Build history of the part. All positions in model axes, mm. A direction names the side the tool comes from. Coordinates: 2 decimals unless noted, no trailing zeros.
(1) Flat gauge pins, fed straight in: P1, Ø6, axis at x = 438, y = 715.5, coming from the -Z side; P2, Ø6.5, axis at x = 301, y = 824.5, coming from the +Z side. Where does each tip first touch, or does it go through?
(2) Wall check: L1, parallel to X at y = 823.5, z = 10. Give the ranges that are in metal, low to high.
(3) Tool access for faces 1 (the face through (296, 685.625, 6)), 2 (the face through (300, 809, 7.7)): list every direction of +Z, -Z, +X, -X, +Y, -Y with a clear straight run to the whole face (end or side of a thin tool).
from build123d import *

# Parameters (mm, degrees)
SKETCH002_W     = 600
SKETCH002_H     = 250
PAD002_DEPTH    = 12.7
SKETCH008_W     = 13
SKETCH008_H     = 264.944031
POCKET002_DEPTH = 5


with BuildPart() as bottom:
    # Sketch002 → Pad002 (new body)
    with BuildSketch(Plane.XY):
        with Locations((300, 541.24469)):
            Rectangle(SKETCH002_W, SKETCH002_H)
    extrude(amount=PAD002_DEPTH)

    # Sketch008 (on Face6 of Pad002) → Pocket002 (cut)
    with BuildSketch(Plane.XY.offset(12.7)):
        with Locations((300, 543.505463)):
            Rectangle(SKETCH008_W, SKETCH008_H)
    extrude(amount=-POCKET002_DEPTH, mode=Mode.SUBTRACT)


with BuildPart() as model_bottom_mirrored:
    # Mirror002: instance of Bottom
    add(bottom.part.mirror(Plane(origin=(-4.230286, 675.934937, 0), x_dir=(-1, 0, 0), z_dir=(0, -1, 0))))


solid = model_bottom_mirrored.part
Response values:
1. P1: stops at z = 0
1. P2: stops at z = 7.7
2. L1: x = 0 to 293.5, 306.5 to 600
3. face 1: +Z, -Z, +X, -X, -Y
3. face 2: +Z, +Y, -Y
